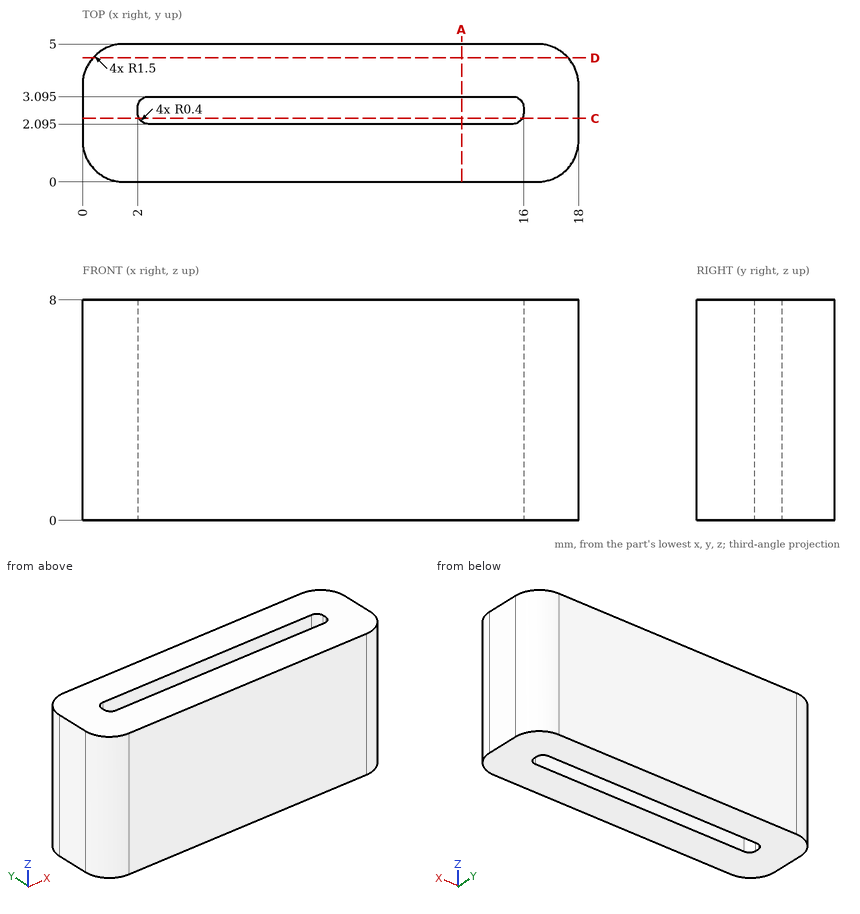
The drawing under review shows one solid part. Ordinate dimensions are in mm from its lowest x, y, z. Coordinates: 2 decimals unless noted, no trailing zeros. Order: outer loops, then holes, each group sorted by start corner. A loop starts at its lowest first (then second) coordinate and runs counter-clockwise, first axis right, second up. Notation, with made-up numbers: (8.5, 21.25) -> (52.5, 21.25) arc R27 cw to (52.5, 56.25) -> close; hole circle Ø10 at (30, -18). An arc over 180 degrees is marked (long way). Answer as CSV lines item,"result".
Q1. Wall thickness on line 1 along Y through (x, z) = (11.25, 2) (1 decimal); line 2 along X through (y, z) = (2.3, 0.5); line 3 along X through (y, z) = (2.8, 4.5) (1 decimal): over which ranges is each line inside the solid? List them lowest first. Write a range as [from, to].
Model answer:
line 1,"y = [0, 2.1], [3.1, 5]"
line 2,"x = [0, 2.05], [15.95, 18]"
line 3,"x = [0, 2], [16, 18]"
Q2. We need section D-D (y = 4.5). State the section outline as (x, z) points, plus the area to 3 significant figures.
Model answer:
outline,"(0.38, 0) -> (17.62, 0) -> (17.62, 8) -> (0.38, 8) -> close"
area,"138 mm2"
Q3. We need section C-C (y = 2.3). State the section outline as (x, z) points.
Model answer:
outline,"(0, 0) -> (2.05, 0) -> (2.05, 8) -> (0, 8) -> close; (15.95, 0) -> (18, 0) -> (18, 8) -> (15.95, 8) -> close"
Q4. We need section A-A (x = 13.75). State the section outline as (y, z) points (1 decimal), plus the area to 3 significant figures.
Model answer:
outline,"(0, 0) -> (2.1, 0) -> (2.1, 8) -> (0, 8) -> close; (3.1, 0) -> (5, 0) -> (5, 8) -> (3.1, 8) -> close"
area,"32.0 mm2"
Q5. Clearance check with a flat-ended pin moving along its axis: pin 1 Ø1.5 at (x, y) = (14.5, 3) entering from -Z. State where the tip first meets the part, or that it passes through.
Model answer:
pin 1,"stops at z = 0"
